Check sheet for the modelled part. Datum: model origin and axes. Units: mm. Face numbers are marked on the shaded views. A direction names the side the tool comes from. Coordinates: 2 decimals unless noted, no trailing zeros. Loops run counter-clockwise (first coordinate to the right, second up) from the corner with the lowest first, then second, coordinate; pieces in that order, holes last. Notation, with made-up numbers: M 67.5,15 L 125.5,15 A33 ccw 125.5,49 Z; hole C 82.25,87 d4. An arc over 180 degrees is marked long. Write each question's results on one line, items separated by ' | '. Start each with the question number.
from build123d import *

# Parameters (mm, degrees)
CYLINDER1798_R     = 3
CYLINDER1798_DEPTH = 20
CYLINDER1796_R     = 2.6
CYLINDER1796_DEPTH = 19
CYLINDER1797_R     = 7.5
CYLINDER1797_DEPTH = 32


with BuildPart() as obj1:
    # Cylinder1798 → Cylinder1798 (new body)
    with BuildSketch(Plane.XY.offset(69)):
        Circle(CYLINDER1798_R)
    extrude(amount=CYLINDER1798_DEPTH)


with BuildPart() as obj2:
    # Cylinder1796 → Cylinder1796 (new body)
    with BuildSketch(Plane.XY.offset(47)):
        Circle(CYLINDER1796_R)
    extrude(amount=CYLINDER1796_DEPTH)


with BuildPart() as cut668:
    # Cylinder1797 → Cylinder1797 (new body)
    with BuildSketch(Plane.XY.offset(50.65)):
        Circle(CYLINDER1797_R)
    extrude(amount=CYLINDER1797_DEPTH)

    # Cut666: cut obj2
    add(obj2.part, mode=Mode.SUBTRACT)

    # Cut668: cut obj1
    add(obj1.part, mode=Mode.SUBTRACT)


solid = cut668.part
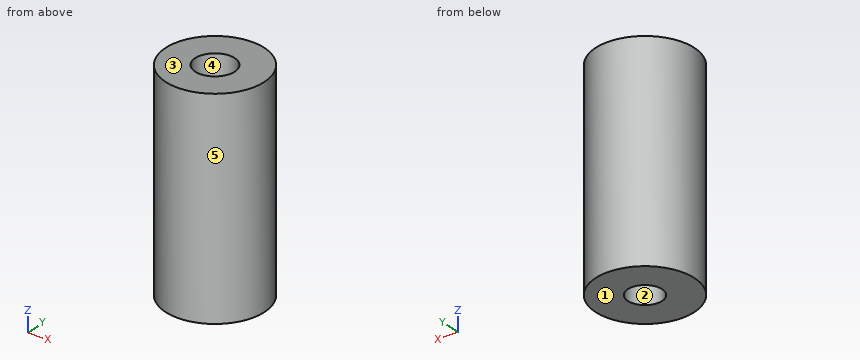
1) Thickness scan on probe 1 along Y at (x, z) = (0, 56.25); probe 2 along Y at (x, z) = (0, 79.5); probe 3 along Y at (x, z) = (-6, 78). Record the ranges inside material, lowest first.
2) Section check D-D (z = 75). Enter the section's corners in (x, y), then the cut area to 3 significant figures.
3) Gauge pin test, flat ends, axial feed: P1, Ø8, axis at y = -2.5, z = 66.5, coming from the -X side; P2, Ø5, axis at x = 0, y = 0, coming from the +Z side; P3, Ø1, axis at y = -6, z = 58.5, coming from the -X side. Record the tip position at first contact, or that the pin passes through.
4) Section check A-A (z = 54). Enter the section's corners in (x, y), then the cut area to 3 significant figures.
5) Section check B-B (x = 0). Enter the section's corners in (y, z).
6) Set-up check for the marked faces 1 and 2: record each of +Z, -Z, +X, -X, +Y, -Y from which the full face is reachable in a straight line by a thin tool's end or side.
7) Release check for a two-part mould opening along X. For the marked faces 3, 4 and 5 record: +X half, -X half, draft (parallel to the pull), parting line (faces both ways), or undercut.
Return value:
1) probe 1: y = -7.5 to -2.6, 2.6 to 7.5 | probe 2: y = -7.5 to -3, 3 to 7.5 | probe 3: y = -4.5 to 4.5
2) outline: C 0,0 d15; hole C 0,0 d6 | area: 148 mm2
3) P1: stops at x = -7.5 | P2: stops at z = 69 | P3: stops at x = -5.1
4) outline: C 0,0 d15; hole C 0,0 d5.2 | area: 155 mm2
5) outline: M -7.5,50.65 L -2.6,50.65 L -2.6,66 L 2.6,66 L 2.6,50.65 L 7.5,50.65 L 7.5,82.65 L 3,82.65 L 3,69 L -3,69 L -3,82.65 L -7.5,82.65 Z
6) face 1: -Z, +X, -X, +Y, -Y | face 2: -Z
7) face 3: draft | face 4: undercut | face 5: parting line
